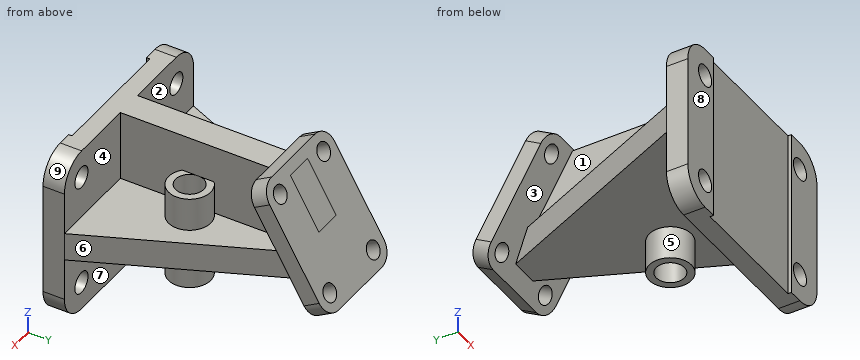
from build123d import *

# Parameters (mm, degrees)
CROQUIS3_W               = 95.25
CROQUIS3_H               = 76.2
SALIENTE_EXTRUIR1_DEPTH  = 9.652
REDONDEO1_R              = 12.7
CROQUIS4_R               = 4.826
CORTAR_EXTRUIR2_DEPTH    = 9.652
CROQUIS6_W               = 12.7
CROQUIS6_H               = 43.017724406
SALIENTE_EXTRUIR3_DEPTH  = 67.564
CROQUIS8_W               = 95.25
CROQUIS8_H               = 12.7
SALIENTE_EXTRUIR4_DEPTH  = 93.218
SALIENTE_EXTRUIR10_DEPTH = 7.874
CORTAR_EXTRUIR8_DEPTH    = 12.7
CROQUIS14_R              = 9.525
SALIENTE_EXTRUIR7_DEPTH  = 14.986
CROQUIS16_R              = 9.525
SALIENTE_EXTRUIR8_DEPTH  = 27.686
CROQUIS17_R              = 6.35
CORTAR_EXTRUIR10_DEPTH   = 60.436
CORTAR_EXTRUIR13_DEPTH   = 12.7
REDONDEO3_R              = 7.874
CROQUIS24_R              = 3.937
CORTAR_EXTRUIR14_DEPTH   = 12.7
CROQUIS25_W              = 12.7
CROQUIS25_H              = 21.99844938
SALIENTE_EXTRUIR11_DEPTH = 31.75
CORTAR_EXTRUIR15_DEPTH   = 31.75
CROQUIS27_W              = 57.404
CROQUIS27_H              = 1.524
CORTAR_EXTRUIR16_DEPTH   = 77.2


with BuildPart() as part:
    # Croquis3 → Saliente-Extruir1 (new body)
    with BuildSketch(Plane(origin=(0, 0, 0), x_dir=(1, 0, 0), z_dir=(0, 1, 0))):
        Rectangle(CROQUIS3_W, CROQUIS3_H)
    extrude(amount=SALIENTE_EXTRUIR1_DEPTH)

    # Redondeo1
    redondeo1_edges = [part.edges().sort_by_distance(p)[0] for p in [
        (47.625, 4.826, 38.1),
        (-47.625, 4.826, 38.1),
        (-47.625, 4.826, -38.1),
        (47.625, 4.826, -38.1),
    ]]
    fillet(redondeo1_edges, radius=REDONDEO1_R)

    # Croquis4 → Cortar-Extruir2 (cut)
    with BuildSketch(Plane(origin=(0, 9.652, 0), x_dir=(1, 0, 0), z_dir=(0, 1, 0))):
        with Locations((-34.925, -25.4)):
            Circle(CROQUIS4_R)
        with Locations((35.052, -25.4)):
            Circle(CROQUIS4_R)
        with Locations((35.052, 25.4)):
            Circle(CROQUIS4_R)
        with Locations((-34.925, 25.4)):
            Circle(CROQUIS4_R)
    extrude(amount=-CORTAR_EXTRUIR2_DEPTH, mode=Mode.SUBTRACT)

    # Croquis6 → Saliente-Extruir3 (add)
    with BuildSketch(Plane(origin=(0, 9.652, 0), x_dir=(1, 0, 0), z_dir=(0, 1, 0))):
        with Locations((0, -16.591137797)):
            Rectangle(CROQUIS6_W, CROQUIS6_H)
    extrude(amount=SALIENTE_EXTRUIR3_DEPTH)

    # Croquis8 → Saliente-Extruir4 (add)
    with BuildSketch(Plane(origin=(0, 9.652, 0), x_dir=(1, 0, 0), z_dir=(0, 1, 0))):
        Rectangle(CROQUIS8_W, CROQUIS8_H)
    extrude(amount=SALIENTE_EXTRUIR4_DEPTH)

    # Croquis11 → Cortar-Extruir8 (cut)
    with BuildSketch(Plane(origin=(0, 0, -6.35), x_dir=(-1, 0, 0), z_dir=(0, 0, -1))):
        Polygon((-6.35, 102.87), (-47.625, 9.652), (-47.625, 102.87), align=None)
    extrude(amount=-CORTAR_EXTRUIR8_DEPTH, mode=Mode.SUBTRACT)

    # Croquis14 → Saliente-Extruir7 (add)
    with BuildSketch(Plane.XY.offset(6.35)):
        with Locations((12.573, 44.704)):
            Circle(CROQUIS14_R)
    extrude(amount=SALIENTE_EXTRUIR7_DEPTH)

    # Croquis16 → Saliente-Extruir8 (add)
    with BuildSketch(Plane.XY.offset(6.35)):
        with Locations((12.573, 44.704)):
            Circle(CROQUIS16_R)
    extrude(amount=-SALIENTE_EXTRUIR8_DEPTH)

    # Croquis17 → Cortar-Extruir10 (cut, through all)
    with BuildSketch(Plane.XY.offset(21.336)):
        with Locations((12.573, 44.704)):
            Circle(CROQUIS17_R)
    extrude(amount=-CORTAR_EXTRUIR10_DEPTH, mode=Mode.SUBTRACT)

    # Croquis13 → Cortar-Extruir13 (cut)
    with BuildSketch(Plane(origin=(0, 0, -6.35), x_dir=(-1, 0, 0), z_dir=(0, 0, -1))):
        Polygon((6.35, 102.87), (47.625, 9.652), (47.625, 102.87), align=None)
    extrude(amount=-CORTAR_EXTRUIR13_DEPTH, mode=Mode.SUBTRACT)



with BuildPart() as body_2:
    # Croquis23 → Saliente-Extruir10 (new body)
    with BuildSketch(Plane(origin=(0, 74.409783942, 42.960508789), x_dir=(1, 0, 0), z_dir=(0, 0.866025404, 0.5))):
        Polygon((0, 5.011636093), (23.876, 5.011636093), (23.876, 65.463636093), (-23.876, 65.463636093), (-23.876, 5.011636093), align=None)
    extrude(amount=SALIENTE_EXTRUIR10_DEPTH)

    # Redondeo3
    redondeo3_edges = [body_2.edges().sort_by_distance(p)[0] for p in [
        (-23.876, 80.325144003, 40.588804619),
        (-23.876, 110.551144003, -11.764163091),
        (23.876, 110.551144003, -11.764163091),
        (23.876, 80.325144003, 40.588804619),
    ]]
    fillet(redondeo3_edges, radius=REDONDEO3_R)

    # Croquis24 → Cortar-Extruir14 (cut)
    with BuildSketch(Plane(origin=(0, 81.228867971, 46.897508789), x_dir=(1, 0, 0), z_dir=(0, 0.866025404, 0.5))):
        with Locations((-16.002, 12.885636093)):
            Circle(CROQUIS24_R)
        with Locations((16.002, 12.885636093)):
            Circle(CROQUIS24_R)
        with Locations((-16.002, 57.589636093)):
            Circle(CROQUIS24_R)
        with Locations((16.002, 57.589636093)):
            Circle(CROQUIS24_R)
    extrude(amount=-CORTAR_EXTRUIR14_DEPTH, mode=Mode.SUBTRACT)


with BuildPart() as part_1:
    add(part.part)

    add(body_2.part)  # Saliente-Extruir11 merges body 2
    # Croquis25 → Saliente-Extruir11 (add)
    with BuildSketch(Plane.XY.offset(6.35)):
        with Locations((0, 88.21522469)):
            Rectangle(CROQUIS25_W, CROQUIS25_H)
    extrude(amount=SALIENTE_EXTRUIR11_DEPTH)

    # Croquis26 → Cortar-Extruir15 (cut)
    with BuildSketch(Plane(origin=(6.35, 0, 0), x_dir=(0, 0, -1), z_dir=(1, 0, 0))):
        Polygon((-15.745567986, 99.21444938), (-38.1, 99.21444938), (-38.1, 86.308112039), align=None)
    extrude(amount=-CORTAR_EXTRUIR15_DEPTH, mode=Mode.SUBTRACT)

    # Croquis27 → Cortar-Extruir16 (cut, through all)
    with BuildSketch(Plane.XY.offset(38.1)):
        with Locations((0, 0.762)):
            Rectangle(CROQUIS27_W, CROQUIS27_H)
    extrude(amount=-CORTAR_EXTRUIR16_DEPTH, mode=Mode.SUBTRACT)


solid = part_1.part
Design review of the part built by this model. Coordinates are the model's own, in mm. Face numbers are marked on the shaded views. A direction names the side the tool comes from. Give positions to 0.01 mm unless a question says otherwise; leave off trailing zeros. Order: outer loops, then holes, each group sorted by start corner. A loop starts at its lowest first (then second) coordinate and runs counter-clockwise, first axis right, second up.
1. Mouldability with a two-part tool opening along Y and no side actions: class the marked faces 6, 7, 8 and 9 as +Y half, -Y half, draft (parallel to the pull), parting line (faces both ways), or undercut.
Solution:
face 6: undercut
face 7: undercut
face 8: -Y half
face 9: draft
2. Add section A-A, the plane x = -18.5. State the section outline as (y, z) points.
Solution:
outline: (1.52, -38.1) - (9.65, -38.1) - (9.65, -6.35) - (75.43, -6.35) - (75.43, 6.35) - (9.65, 6.35) - (9.65, 38.1) - (1.52, 38.1) - close; (77.12, 38.27) - (79.33, 34.44) - (86.15, 38.37) - (83.94, 42.21) - close; (82.37, 29.17) - (101.68, -4.28) - (108.5, -0.34) - (89.19, 33.1) - close; (104.73, -9.55) - (106.94, -13.38) - (113.76, -9.44) - (111.55, -5.61) - close
3. To check wall thickness, follow L1, parallel to X at y = 6.75, z = -25.4 (3 decimals); L2, parallel to X at y = 2, z = -25 (3 decimals); L3, parallel to X at y = 46.5, z = 37.5. State the ranges of each line that lie inside material, in increasing order.
Solution:
L1: x = -47.625 to -39.751, -30.099 to 30.226, 39.878 to 47.625
L2: x = -47.625 to -39.734, -30.116 to 30.243, 39.861 to 47.625
L3: x = -6.35 to 6.35
4. Add section C-C, the plane z = 4. State the section outline as (x, y) points (3 decimals).
Solution:
outline: (-47.625, 0) - (-28.702, 0) - (-28.702, 1.524) - (28.702, 1.524) - (28.702, 0) - (47.625, 0) - (47.625, 9.652) - (8.992, 96.904) - (23.876, 96.904) - (23.876, 105.996) - (-23.876, 105.996) - (-23.876, 96.904) - (-8.992, 96.904) - (-47.625, 9.652) - close; hole circle Ø12.7 at (12.573, 44.704)
5. Tool access review of the marked faces 1, 2, 3, 4 and 5: name each direction out of +Z, -Z, +X, -X, +Y, -Y from which nothing blocks a thin tool from reaching the whole face with its end or side.
Solution:
face 1: -X
face 2: +Z, -X
face 3: none
face 4: +Z, +X
face 5: -Z
6. For pin 1 Ø12 at (x, z) = (22.5, -28.5) entering from +Y; pin 2 Ø9.5 at (x, z) = (19, -15) entering from +Y; pin 3 Ø1 at (y, z) = (82.5, 26) entering from -X; pin 4 Ø12.5 at (x, y) = (-35, 59.5) entering from +Z, all flat-tipped, find the tip position at first contact; note any pin that passes through.
Solution:
pin 1: stops at y = 9.65
pin 2: stops at y = 112.49
pin 3: stops at x = -6.35
pin 4: passes through
7. Add section B-B, the plane y = 65. State the section outline as (x, z) points, then the cut area to 3 significant figures.
Solution:
outline: (-23.12, -6.35) - (23.12, -6.35) - (23.12, 6.35) - (6.35, 6.35) - (6.35, 38.1) - (-6.35, 38.1) - (-6.35, 6.35) - (-23.12, 6.35) - close
area: 990 mm2
